Design review of the part built by this model. Coordinates are the model's own, in mm. A direction names the side the tool comes from. Coordinates: 2 decimals unless noted, no trailing zeros. Loops run counter-clockwise (first coordinate to the right, second up) from the corner with the lowest first, then second, coordinate; pieces in that order, holes last. Notation, with made-up numbers: (33, 77) -> (71, 77) arc R25 ccw to (71, 100) -> close; hole circle Ø5 at (42.5, 6). An arc over 180 degrees is marked (long way). Use one line per item in the form item = value. Start each with the question number.
1. For pin 1 (3 mm diameter, centred on x = -3.5, y = 6, fed in from -Z), flat-tipped, find the tip position at first contact; note if it passes through.
2. The part is to be moulded in two halves that separate along X. For faces 3 (the face through (57.9, 5, 1)), 4 (the face through (1, 5, 2)), 5 (the face through (-23.15, 10, 1)), say which applies: released by +X, released by -X, zero draft, split by the parting line, or undercut.
3. Consider section A-A (y = 10). State the section outline as (x, z) points, then the cut area to 3 significant figures.
4. Wall thickness on line 1 (X direction, y = 5.5, z = 1.2); line 2 (X direction, y = 12, z = 1.25); line 3 (Y direction, x = -13.5, z = 0.8): over which ranges is each line inside the solid? List them lowest first. Write a range as from..to.
5. Consider section B-B (z = 1.25). State how many separate pieces and enclosed holes the cut face has, then the cut area to 3 significant figures.
6. Machinability: for faces 1 (the face through (-1, 36.8, 1)), 2 (the face through (-21, -11.4, 1)), which of the approach directions +Z, -Z, +X, -X, +Y, -Y give a long, thin tool a straight path to every point of the face, cutting with its end or side? Answer none if there is none.
from build123d import *

# Parameters (mm, degrees)
SKETCH1_W           = 105.8
SKETCH1_H           = 53.6
BOSS_EXTRUDE1_DEPTH = 2
SKETCH2_W           = 4.1
SKETCH2_H           = 7.1
SKETCH2_W_2         = 20.5
SKETCH2_H_2         = 13.5
SKETCH2_W_3         = 10
SKETCH2_H_3         = 10
SKETCH2_W_4         = 7.1
SKETCH2_W_5         = 14
SKETCH2_W_6         = 10.1
CUT_EXTRUDE2_DEPTH  = 60.335065518
SKETCH4_W           = 2.5
SKETCH4_H           = 2.7
SKETCH4_W_2         = 1.75
SKETCH4_H_2         = 3.6
SKETCH4_W_3         = 1.7
SKETCH4_H_3         = 1.3
SKETCH4_W_4         = 10.6
SKETCH4_H_4         = 8.4
SKETCH4_W_5         = 3.5
SKETCH4_H_5         = 11.1
SKETCH4_W_6         = 14.5
SKETCH4_H_6         = 5
CUT_EXTRUDE5_DEPTH  = 10
BOSS_EXTRUDE2_DEPTH = 2


with BuildPart() as part:
    # Sketch1 → Boss-Extrude1 (new body)
    with BuildSketch(Plane.XY):
        Rectangle(SKETCH1_W, SKETCH1_H)
    extrude(amount=BOSS_EXTRUDE1_DEPTH)

    # Sketch2 → Cut-Extrude2 (cut, through all)
    with BuildSketch(Plane.XY):
        with Locations((11.65, -10.05)):
            Rectangle(SKETCH2_W, SKETCH2_H)
        with Locations((-32.65, -10.05)):
            Rectangle(SKETCH2_W_2, SKETCH2_H_2)
        with Locations((24.75, 10.05)):
            Rectangle(SKETCH2_W_3, SKETCH2_H_3)
        with Locations((39.35, -10.05)):
            Rectangle(SKETCH2_W_4, SKETCH2_H)
        with Locations((-32.65, 10.05)):
            Rectangle(SKETCH2_W_5, SKETCH2_H_2)
        with Locations((24.75, -10.05)):
            Rectangle(SKETCH2_W_4, SKETCH2_H)
        with Locations((-7.35, -10.05)):
            Rectangle(SKETCH2_W_6, SKETCH2_H)
    extrude(amount=CUT_EXTRUDE2_DEPTH, mode=Mode.SUBTRACT)

    # Sketch4 → Cut-Extrude5 (cut)
    with BuildSketch(Plane.XY.offset(2)):
        with Locations((-24.4, 10.05)):
            Rectangle(SKETCH4_W, SKETCH4_H)
        with Locations((-40.9, 10.05)):
            Rectangle(SKETCH4_W, SKETCH4_H)
        with Locations((-44.15, -10.05)):
            Rectangle(SKETCH4_W, SKETCH4_H)
        with Locations((-21.15, -10.05)):
            Rectangle(SKETCH4_W, SKETCH4_H)
        with Locations((-13.275, -10.05)):
            Rectangle(SKETCH4_W_2, SKETCH4_H_2)
        with Locations((-1.425, -10.05)):
            Rectangle(SKETCH4_W_2, SKETCH4_H_2)
        with Locations((-7.35, -5.85)):
            Rectangle(SKETCH4_W_3, SKETCH4_H_3)
        with Locations((11.65, -5.85)):
            Rectangle(SKETCH4_W_3, SKETCH4_H_3)
        with Locations((14.575, -10.05)):
            Rectangle(SKETCH4_W_2, SKETCH4_H_2)
        with Locations((8.725, -10.05)):
            Rectangle(SKETCH4_W_2, SKETCH4_H_2)
        with Locations((29.175, -10.05)):
            Rectangle(SKETCH4_W_2, SKETCH4_H_2)
        with Locations((20.325, -10.05)):
            Rectangle(SKETCH4_W_2, SKETCH4_H_2)
        with Locations((24.75, -5.85)):
            Rectangle(SKETCH4_W_3, SKETCH4_H_3)
        with Locations((39.35, -10.05)):
            Rectangle(SKETCH4_W_4, SKETCH4_H_2)
        with Locations((39.35, -9.4)):
            Rectangle(SKETCH4_W_3, SKETCH4_H_4)
        with Locations((24.75, 10.6)):
            Rectangle(SKETCH4_W_5, SKETCH4_H_5)
        with Locations((24.75, 10.05)):
            Rectangle(SKETCH4_W_6, SKETCH4_H_6)
    extrude(amount=-CUT_EXTRUDE5_DEPTH, mode=Mode.SUBTRACT)

    # Sketch5 → Boss-Extrude2 (add)
    with BuildSketch(Plane.XY):
        Polygon((-52.9, 26.8), (-52.9, -26.8), (-57.9, -26.8), (-57.9, 36.8), (57.9, 36.8), (57.9, -26.8), (52.9, -26.8), (52.9, 26.8), align=None)
    extrude(amount=BOSS_EXTRUDE2_DEPTH)


solid = part.part
Geometry check:
q1.pin_1 = 0
q2.face_3 = released by +X
q2.face_4 = zero draft
q2.face_5 = undercut
q3.outline = (-57.9, 0) -> (-42.15, 0) -> (-42.15, 2) -> (-57.9, 2) -> close; (-23.15, 0) -> (17.5, 0) -> (17.5, 2) -> (-23.15, 2) -> close; (32, 0) -> (57.9, 0) -> (57.9, 2) -> (32, 2) -> close
q3.area = 165 mm²
q4.line_1 = -57.9..-39.65, -25.65..19.75, 29.75..57.9
q4.line_2 = -57.9..-39.65, -25.65..17.5, 32..57.9
q4.line_3 = -26.8..-11.85, -8.25..36.8
q5.separate_pieces = 1
q5.enclosed_holes = 7
q5.area = 6,480 mm²
q6.face_1 = +Z, -Z, +X, -X, +Y
q6.face_2 = +Z, -Z
